```python
from build123d import *

# Parameters (mm, degrees)
SKETCH1_R           = 1.3462
SKETCH1_W           = 60.6932
SKETCH1_H           = 7.81
SKETCH1_W_2         = 5.588
SKETCH1_H_2         = 23.368
SKETCH1_W_3         = 5.4034
SKETCH1_H_3         = 22.6066
BOSS_EXTRUDE1_DEPTH = 3.048
SKETCH2_R           = 10.922
SKETCH2_R_2         = 1.4986
CUT_EXTRUDE1_DEPTH  = 4.048
SKETCH3_W           = 60.6932
SKETCH3_H           = 56.8638
BOSS_EXTRUDE2_DEPTH = 3.048


with BuildPart() as part:
    # Sketch1 → Boss-Extrude1 (new body)
    with BuildSketch(Plane.XY):
        with BuildLine():
            Line((61.214907375, 24.068294304), (40.134807375, 24.068294304))
            Line((40.134807375, 24.068294304), (40.134807375, 8.658194304))
            Line((40.134807375, 8.658194304), (56.975007375, 8.658194304))
            Line((56.975007375, 8.658194304), (56.975007375, 4.997894304))
            Line((56.975007375, 4.997894304), (40.134807375, 4.997894304))
            Line((40.134807375, 4.997894304), (40.134807375, -9.121805696))
            Line((40.134807375, -9.121805696), (56.975007375, -9.121805696))
            Line((56.975007375, -9.121805696), (56.975007375, -12.628005696))
            Line((56.975007375, -12.628005696), (35.575007375, -12.628005696))
            Line((35.575007375, -12.628005696), (35.575007375, -28.627805696))
            Line((35.575007375, -28.627805696), (61.214907375, -28.627805696))
            Line((61.214907375, -28.627805696), (61.214907375, -32.613401529))
            ThreePointArc((61.214907375, -32.613401529), (60.108826144, -35.325305244), (57.405007375, -36.451005696))
            Line((57.405007375, -36.451005696), (38.714307375, -36.451005696))
            Line((38.714307375, -36.451005696), (28.474307375, -33.084405696))
            Line((28.474307375, -33.084405696), (-23.844892625, -33.084405696))
            Line((-23.844892625, -33.084405696), (-34.084892625, -36.451005696))
            ThreePointArc((-34.084892625, -36.451005696), (-36.778969461, -35.335082532), (-37.894892625, -32.641005696))
            Line((-37.894892625, -32.641005696), (-37.894892625, 26.697694304))
            ThreePointArc((-37.894892625, 26.697694304), (-36.778969461, 29.391771141), (-34.084892625, 30.507694304))
            Line((-34.084892625, 30.507694304), (57.404932375, 30.507694304))
            ThreePointArc((57.404932375, 30.507694304), (60.103884597, 29.386886916), (61.214907375, 26.683892153))
            Line((61.214907375, 26.683892153), (61.214907375, 24.068294304))
        make_face()
        with Locations((57.404932375, 26.697694304)):
            Circle(SKETCH1_R, mode=Mode.SUBTRACT)
        with Locations((-34.084892625, 26.697694304)):
            Circle(SKETCH1_R, mode=Mode.SUBTRACT)
        with Locations((-34.084892625, -32.641005696)):
            Circle(SKETCH1_R, mode=Mode.SUBTRACT)
        with Locations((57.405007375, -32.641005696)):
            Circle(SKETCH1_R, mode=Mode.SUBTRACT)
        with Locations((1.341707375, 21.991994304)):
            Rectangle(SKETCH1_W, SKETCH1_H, mode=Mode.SUBTRACT)
        with Locations((-26.210892625, -1.882805696)):
            Rectangle(SKETCH1_W_2, SKETCH1_H_2, mode=Mode.SUBTRACT)
        with Locations((16.546707375, -19.663505696)):
            Rectangle(SKETCH1_W_3, SKETCH1_H_3, mode=Mode.SUBTRACT)
    extrude(amount=BOSS_EXTRUDE1_DEPTH)

    # Sketch2 → Cut-Extrude1 (cut, through all)
    with BuildSketch(Plane.XY.offset(3.048)):
        with Locations((-0.302892625, -0.480305696)):
            Circle(SKETCH2_R)
        with Locations((-10.285092625, -10.462505696)):
            Circle(SKETCH2_R_2)
        with Locations((-10.285092625, 9.501894304)):
            Circle(SKETCH2_R_2)
        with Locations((9.679307375, -10.462505696)):
            Circle(SKETCH2_R_2)
        with Locations((9.679307375, 9.501894304)):
            Circle(SKETCH2_R_2)
    extrude(amount=-CUT_EXTRUDE1_DEPTH, mode=Mode.SUBTRACT)

    # Sketch3 → Boss-Extrude2 (add)
    with BuildSketch(Plane.XY.offset(3.048)):
        with Locations((1.341707375, -2.534905696)):
            Rectangle(SKETCH3_W, SKETCH3_H)
    extrude(amount=-BOSS_EXTRUDE2_DEPTH)


solid = part.part
```
The model under review builds one solid part; all positions refer to its coordinate system, in mm. A direction names the side the tool comes from. Round coordinates to 2 decimals unless told otherwise and drop trailing zeros. Write each loop counter-clockwise with the first axis right and the second up, starting at its lowest first coordinate (ties: lowest second). Pieces come first, ordered by that corner, then holes. Notation, with made-up numbers: (84.25, 31) -> (130.25, 31) arc R4 ccw to (130.25, 35) -> close; hole circle Ø3 at (68, 21). An arc over 180 degrees is marked (long way). Use CSV: the item, a comma, the result in double quotes.
Q1. Consider section A-A (z = 2.15). Give the boundary of the cut face in (x, y) (3 decimals), then the cut area to 3 significant figures.
Checks:
outline,"(-37.895, -32.641) arc R3.81 ccw to (-34.085, -36.451) -> (-23.845, -33.084) -> (28.474, -33.084) -> (38.714, -36.451) -> (57.405, -36.451) arc R3.81 ccw to (61.215, -32.613) -> (61.215, -28.628) -> (35.575, -28.628) -> (35.575, -12.628) -> (56.975, -12.628) -> (56.975, -9.122) -> (40.135, -9.122) -> (40.135, 4.998) -> (56.975, 4.998) -> (56.975, 8.658) -> (40.135, 8.658) -> (40.135, 24.068) -> (61.215, 24.068) -> (61.215, 26.684) arc R3.81 ccw to (57.405, 30.508) -> (-34.085, 30.508) arc R3.81 ccw to (-37.895, 26.698) -> close; hole circle Ø2.692 at (-34.085, -32.641); hole circle Ø2.692 at (-34.085, 26.698); hole circle Ø2.692 at (57.405, -32.641); hole circle Ø2.692 at (57.405, 26.698)"
area,"5,330 mm²"
Q2. For faces 5 (the cylindrical face through (-35.43, 26.76, 1.5)), 6 (the flat face through (46, -12.628, 2)), list the 3-axis set-ups (+Z, -Z, +X, -X, +Y, -Y) from which the entire face can be reached by the end or side of a thin tool; tool diameter is ignored.
Checks:
face 5,"+Z, -Z"
face 6,"+Z, -Z, +X"
Q3. Consider section B-B (y = -7). Give the boundary of the cut face in (x, z), then the cut area to 3 significant figures.
Checks:
outline,"(-37.89, 0) -> (40.13, 0) -> (40.13, 3.05) -> (-37.89, 3.05) -> close"
area,"238 mm²"
Q4. To check wall thickness, follow probe 1 along Y at (x, z) = (46, 1.7); probe 2 along X at (y, z) = (9.5, 1.85); probe 3 along Y at (x, z) = (8, 1.65). State the ranges of each line that lie inside material, in increasing order. Write a range as [from, to].
Checks:
probe 1,"[-36.45, -28.63], [-12.63, -9.12], [5, 8.66], [24.07, 30.51]"
probe 2,"[-37.89, 40.13]"
probe 3,"[-33.08, 30.51]"
Q5. For pin 1 Ø2 at (x, y) = (57.41, -32.64) entering from -Z; pin 2 Ø1.5 at (x, z) = (5, 1.5) entering from -Y; pin 3 Ø1.5 at (y, z) = (18.5, 1) entering from +X, all flat-tipped, find the tip position at first contact; note any pin that passes through.
Checks:
pin 1,"through"
pin 2,"y = -33.08"
pin 3,"x = 40.13"
Q6. Consider section C-C (x = -3). Give the boundary of the cut face in (y, z).
Checks:
outline,"(-33.08, 0) -> (30.51, 0) -> (30.51, 3.05) -> (-33.08, 3.05) -> close"
Q7. Mouldability with a two-part tool opening along Y and no side actions: class faces 1 (the flat face through (51, 24.068, 2)), 2 (the flat face through (1, -3, 3.048)), 3 (the flat face through (3, -33.084, 2)), 4 (the cylindrical face through (56.06, -32.58, 1.5)) as released by +Y, released by -Y, zero draft, split by the parting line, or undercut.
Checks:
face 1,"undercut"
face 2,"zero draft"
face 3,"released by -Y"
face 4,"undercut"
